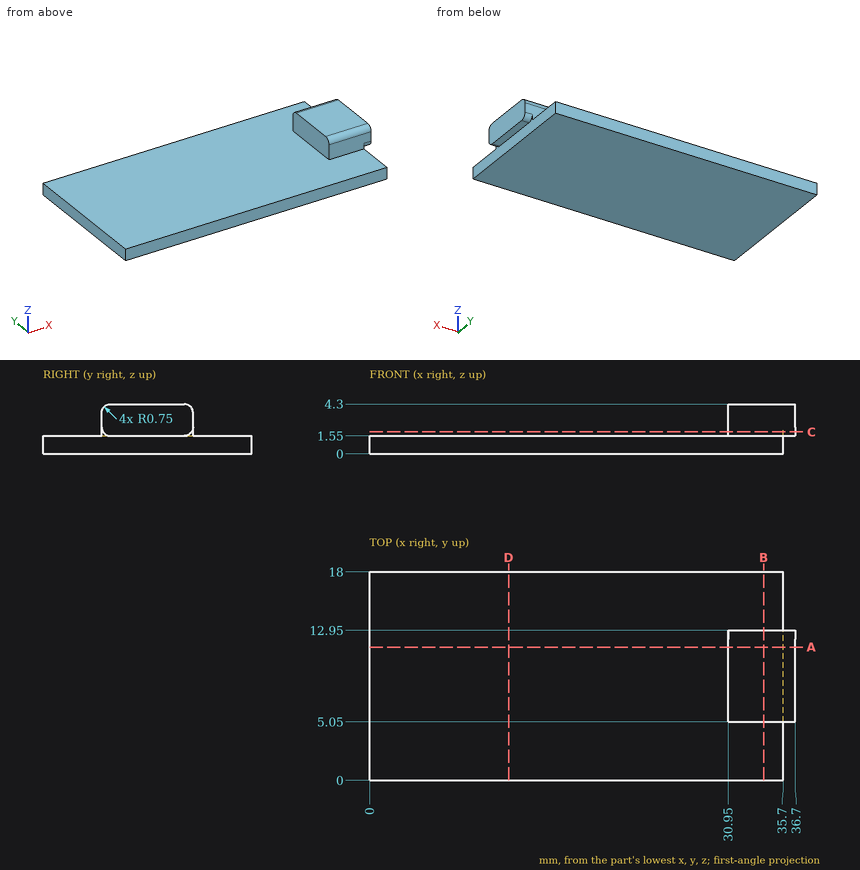
Design review of the part shown in the three views and the two pictorial views. Dimensions are in mm from the part's minimum x, y and z. Round coordinates to 2 decimals unless told otherwise and drop trailing zeros. Write each loop counter-clockwise with the first axis right and the second up, starting at its lowest first coordinate (ties: lowest second). Pieces come first, ordered by that corner, then holes.
Item 1: Consider section B-B on x = 34. Give the boundary of the cut face in (y, z), and give its area (3 significant figures).
Item 2: Wall thickness on L1, parallel to X at y = 8.5, z = 1.1; L2, parallel to Z at x = 12, y = 1.5; L3, parallel to X at y = 10, z = 3.05: over which ranges is each line inside the solid? List them lowest first.
Item 3: Consider section A-A on y = 11.5. Give the boundary of the cut face in (x, z).
Item 4: Consider section D-D on x = 12. Give the boundary of the cut face in (y, z), and give its area (3 significant figures).
Item 5: For pin 1 Ø1.5 at (x, y) = (18, 3.5) entering from +Z; pin 2 Ø1.4 at (y, z) = (7.5, 2.5) entering from -X; pin 3 Ø1.6 at (x, z) = (34, 3) entering from +Y, all flat-tipped, find the tip position at first contact; note any pin that passes through.
Item 6: Consider section C-C on z = 1.9. Give the boundary of the cut face in (x, y).
Check values:
1. outline: (0, 0) - (18, 0) - (18, 1.55) - (12.95, 1.55) - (12.95, 3.55) arc R0.75 ccw to (12.2, 4.3) - (5.8, 4.3) arc R0.75 ccw to (5.05, 3.55) - (5.05, 1.55) - (0, 1.55) - close
1. area: 49.4 mm2
2. L1: x = 0 to 35.7
2. L2: z = 0 to 1.55
2. L3: x = 30.95 to 36.7
3. outline: (0, 0) - (35.7, 0) - (35.7, 1.55) - (36.7, 1.55) - (36.7, 4.3) - (30.95, 4.3) - (30.95, 1.55) - (0, 1.55) - close
4. outline: (0, 0) - (18, 0) - (18, 1.55) - (0, 1.55) - close
4. area: 27.9 mm2
5. pin 1: stops at z = 1.55
5. pin 2: stops at x = 30.95
5. pin 3: stops at y = 12.95
6. outline: (30.95, 5.05) - (35.7, 5.05) - (35.7, 5.17) - (36.7, 5.17) - (36.7, 12.83) - (35.7, 12.83) - (35.7, 12.95) - (30.95, 12.95) - close
